```python
from build123d import *

# Parameters (mm, degrees)
SKETCH1_R           = 6.35
BOSS_EXTRUDE1_DEPTH = 25.4
SHELL1_T            = -0.889
FILLET1_R           = 1.27
SKETCH2_R           = 4.7625
BOSS_EXTRUDE2_DEPTH = 10.16
CUT_EXTRUDE1_START  = -10.16
CUT_EXTRUDE1_DEPTH  = 10.16
SKETCH4_R           = 3.048
CUT_EXTRUDE2_DEPTH  = 28.452277251
FILLET2_R           = 0.381
FILLET3_R           = 1.27


with BuildPart() as part:
    # Sketch1 → Boss-Extrude1 (new body)
    with BuildSketch(Plane.XY):
        Circle(SKETCH1_R)
    extrude(amount=BOSS_EXTRUDE1_DEPTH)

    # Shell1
    shell1_openings = [part.faces().sort_by_distance(p)[0] for p in [
        (0, 0, 25.4),
    ]]
    offset(amount=SHELL1_T, openings=shell1_openings, kind=Kind.INTERSECTION)

    # Fillet1
    fillet1_edges = [part.edges().sort_by_distance(p)[0] for p in [
        (-6.35, 0, 0),
    ]]
    fillet(fillet1_edges, radius=FILLET1_R)

    # Sketch2 → Boss-Extrude2 (add)
    with BuildSketch(Plane(origin=(0, 0, 0), x_dir=(-1, 0, 0), z_dir=(0, 0, -1))):
        with Locations(Location((0, 0, 0), (0, 0, 180))):
            Circle(SKETCH2_R)
    extrude(amount=BOSS_EXTRUDE2_DEPTH)

    # Sketch3 → Cut-Extrude1 (cut)
    with BuildSketch(Plane(origin=(0, 0, -10.16), x_dir=(-1, 0, 0), z_dir=(0, 0, -1)).offset(CUT_EXTRUDE1_START)):
        with BuildLine():
            Line((-1.905, 4.364903349), (-1.905, -4.364903349))
            ThreePointArc((-1.905, -4.364903349), (-4.7625, 0), (-1.905, 4.364903349))
        make_face()
        with BuildLine():
            Line((1.905, 4.364903349), (1.905, -4.364903349))
            ThreePointArc((1.905, -4.364903349), (4.7625, 0), (1.905, 4.364903349))
        make_face()
    extrude(amount=CUT_EXTRUDE1_DEPTH, mode=Mode.SUBTRACT)

    # Sketch4 → Cut-Extrude2 (cut, through all)
    with BuildSketch(Plane(origin=(1.905, 0, 0), x_dir=(0, 0, -1), z_dir=(1, 0, 0))):
        with Locations((5.3975, 0)):
            Circle(SKETCH4_R)
    extrude(amount=-CUT_EXTRUDE2_DEPTH, mode=Mode.SUBTRACT)

    # Fillet2
    fillet2_edges = [part.edges().sort_by_distance(p)[0] for p in [
        (-1.905, 0, -2.3495),
        (1.905, 0, -2.3495),
    ]]
    fillet(fillet2_edges, radius=FILLET2_R)

    # Fillet3
    fillet3_edges = [part.edges().sort_by_distance(p)[0] for p in [
        (0, 4.7625, -10.16),
        (0, -4.7625, -10.16),
    ]]
    fillet(fillet3_edges, radius=FILLET3_R)


solid = part.part
```
The model under review builds one solid part; all positions refer to its coordinate system, in mm. A direction names the side the tool comes from. Round coordinates to 2 decimals unless told otherwise and drop trailing zeros. Loops run counter-clockwise (first coordinate to the right, second up) from the corner with the lowest first, then second, coordinate; pieces in that order, holes last. Notation, with made-up numbers: M -6.5,7 L 21.5,7 A6 ccw 21.5,17 Z; hole C -30,67 d9. An arc over 180 degrees is marked long. Put each result on its own line as item: value.
Q1. For pin 1 (5 mm diameter, centred on y = -2, z = -1.5, fed in from -X); pin 2 (1 mm diameter, centred on y = -4, z = 14.5, fed in from +X); pin 3 (1.5 mm diameter, centred on x = 1.5, z = 20, fed in from +Y), all flat-tipped, find the tip position at first contact; note any pin that passes through.
Result set:
pin 1: stops at x = -6.18
pin 2: stops at x = 5.3
pin 3: stops at y = 6.31
Q2. To check wall thickness, follow L1, parallel to Y at x = 0, z = 6.75; L2, parallel to X at y = -3.5, z = 7.5; L3, parallel to Z at x = -2.5, y = 2.5. State the ranges of each line that lie inside material, in increasing order.
Result set:
L1: y = -6.35 to -5.46, 5.46 to 6.35
L2: x = -5.3 to -4.19, 4.19 to 5.3
L3: z = 0 to 0.89
Q3. Consider section A-A, the plane x = 0. Give the boundary of the cut face in (y, z), then the cut area to 3 significant figures.
Result set:
outline: M -6.35,1.27 A1.27 ccw -5.08,0 L -4.76,0 L -4.76,-8.89 A1.27 ccw -3.49,-10.16 L 3.49,-10.16 A1.27 ccw 4.76,-8.89 L 4.76,0 L 5.08,0 A1.27 ccw 6.35,1.27 L 6.35,25.4 L 5.46,25.4 L 5.46,0.89 L -5.46,0.89 L -5.46,25.4 L -6.35,25.4 Z; hole C 0,-5.4 d6.1
area: 121 mm²
Q4. Consider section C-C, the plane z = 15. Give the boundary of the cut face in (x, y), then the cut area to 3 significant figures.
Result set:
outline: C 0,0 d12.7; hole C 0,0 d10.92
area: 33.0 mm²
Q5. Mouldability with a two-part tool opening along Y and no side actions: class faces 1 (the flat face through (0, 0, 0.889)), 2 (the cylindrical face through (-1.38, -6.2, 13.17)), 3 (the flat face through (-1.905, 0.1, -1.6)) as released by +Y, released by -Y, zero draft, split by the parting line, or undercut.
Result set:
face 1: undercut
face 2: split by the parting line
face 3: zero draft
Q6. Machinability: for faces 4 (the cylindrical face through (-0.027, 4.762, -4.383)), 5 (the cylindrical face through (0.027, -4.762, -4.383)), 6 (the cylindrical face through (5.21, 1.64, 12.97)), which of the approach directions +Z, -Z, +X, -X, +Y, -Y give a long, thin tool a straight path to every point of the face, cutting with its end or side? Answer none if there is none.
Result set:
face 4: -Z, +Y
face 5: -Z, -Y
face 6: +Z
